Autodesk Inventor part; units mm, degrees
ref_plane "YZ Plane" through (0, 0, 0) normal (1, 0, 0) x (0, 1, 0)
ref_plane "XZ Plane" through (0, 0, 0) normal (0, 1, 0) x (-1, 0, 0)
ref_plane "XY Plane" through (0, 0, 0) normal (0, 0, 1) x (1, 0, 0)
sketch "Sketch1" plane through (0, 0, 0) normal (0, 1, 0) x (-1, 0, 0)
  line L0 (-15, -15) -> (15, -15)
  line L1 (15, -15) -> (15, 15)
  line L2 (15, 15) -> (-15, 15)
  line L3 (-15, 15) -> (-15, -15)
  line L4 (-15, -15) -> (15, 15) construction
  line L5 (15, -15) -> (-15, 15) construction
  point P0 (0, 0)
  dimension "d0" = 30
  dimension "d1" = 30
extrude "Extrusion1" add sketch "Sketch1" along normal blind 5
sketch "Sketch2" plane through (15, 0, 15) normal (1, 0, 0) x (0, 0, -1)
  line L0 (0, 5) -> (30, 5)
  line L1 (5, 4.05) -> (25, 4.05)
  line L2 (0, 0) -> (30, 0)
  line L3 (5, 4.6) -> (5, 4.05)
  line L4 (5, 4.6) -> (6, 4.6)
  line L5 (6, 4.6) -> (6, 5)
  line L6 (15, -1.7486) -> (15, 8.5822)
  line L7 (25, 4.05) -> (5, 4.05)
  line L8 (25, 4.6) -> (25, 4.05)
  line L9 (25, 4.6) -> (24, 4.6)
  line L10 (24, 4.6) -> (24, 5)
  point P0 (15, 0)
  point P1 (15, 0)
  point P2 (15, 0)
  dimension "d4" = 10
  dimension "d5" = 20
  dimension "d10" = 0.55
  dimension "d12" = 0.4
  dimension "d13" = 1
extrude "Extrusion2" cut sketch "Sketch2" against normal blind 25
sketch "Sketch3" plane through (0, 5, 0) normal (0, 1, 0) x (1, 0, 0)
  line L0 (-10, 9) -> (15, 9)
  line L1 (15, -9) -> (-10, -9)
  line L2 (-10, 9) -> (-7.5, 9)
  line L3 (-7.5, 9) -> (-7.5, -9)
  line L4 (-7.5, -9) -> (-10, -9)
  line L5 (-10, -9) -> (-10, 9)
  line L6 (-7.5, -1) -> (-10, -1)
  line L7 (-10, -1) -> (-10, 1)
  line L8 (-10, 1) -> (-7.5, 1)
  line L9 (-7.5, 1) -> (-7.5, -1)
  point P0 (0, 0)
  dimension "d16" = 2.5
  dimension "d17" = 2
  dimension "d18" = 1
extrude "Extrusion3" add sketch "Sketch3" against normal up to surface (0.4 mm away) contours L0 L3 L8 L5 | L6 L3 L1 L5
fillet "Fillet1" radius 1 6 edges at (15, 4.8, 9) (15, 4.8, -9) (-7.5, 4.8, -1) (-7.5, 4.8, 1) (-7.5, 4.8, 9) (-7.5, 4.8, -9)
sketch "Sketch4" plane through (0, 5, 0) normal (0, 1, 0) x (1, 0, 0)
  point P0 (0, 0)
  point P1 (12.5, -12.5)
  point P2 (-12.5, -12.5)
  point P3 (-12.5, 12.5)
  point P4 (12.5, 12.5)
  dimension "d22" = 25
  dimension "d23" = 12.5
  dimension "d24" = 25
  dimension "d25" = 12.5
hole "Hole1" at (12.5, 5, 12.5) at (-12.5, 5, 12.5) at (-12.5, 5, -12.5) at (12.5, 5, -12.5) direction (0, -1, 0) diameter 2 end through all
properties part number "Flex Circuit Slot"
For this review, take the finished solid that the model builds, in its own axes (mm). A direction names the side the tool comes from. Round coordinates to 2 decimals unless told otherwise and drop trailing zeros. Write each loop counter-clockwise with the first axis right and the second up, starting at its lowest first coordinate (ties: lowest second). Pieces come first, ordered by that corner, then holes. Notation, with made-up numbers: (6.25, 6.5) - (37.25, 6.5) arc R13 ccw to (37.25, 22.5) - close; hole circle Ø7 at (87, -14). An arc over 180 degrees is marked (long way). Use a Markdown table: item, result.
Q1. We need section A-A (x = -12.5). Give the boundary of the cut face in (y, z).
Derived:
| item | result |
|---|---|
| outline | (0, -15) - (5, -15) - (5, -13.5) - (0, -13.5) - close; (0, -11.5) - (5, -11.5) - (5, 11.5) - (0, 11.5) - close; (0, 13.5) - (5, 13.5) - (5, 15) - (0, 15) - close |
Q2. Wall thickness on line 1 along X through (y, z) = (3.3, 12.5); line 2 along Z through (x, y) = (-4.75, 4.25): over which ranges is each line inside the solid? List them lowest first.
Derived:
| item | result |
|---|---|
| line 1 | x = -15 to -13.5, -11.5 to 11.5, 13.5 to 15 |
| line 2 | z = -15 to -10, 10 to 15 |
Q3. We need section B-B (z = 3.25). Give the boundary of the cut face in (x, y), plus the area to 3 significant figures.
Derived:
| item | result |
|---|---|
| outline | (-15, 0) - (15, 0) - (15, 4.05) - (-10, 4.05) - (-10, 4.6) - (-7.5, 4.6) - (-7.5, 5) - (-15, 5) - close |
| area | 127 mm2 |
Q4. The part is to be moulded in two halves that separate along Z. For faces 1 (the flat face through (-10, 5, 4)), 2 (the flat face through (0, 2, 15)), 3 (the cylindrical face through (-7.199, 4.797, 8.715)), say which applies: pulls with the +Z half, pulls with the -Z half, needs draft (parallel to the pull), parting line crosses it, or undercut.
Derived:
| item | result |
|---|---|
| face 1 | needs draft |
| face 2 | pulls with the +Z half |
| face 3 | undercut |
Q5. Clearance check with a flat-ended pin moving along its axis: pin 1 (1 mm diameter, centred on x = 3.5, z = -2.5, fed in from +Y). State where the tip first meets the part, or that it passes through.
Derived:
| item | result |
|---|---|
| pin 1 | stops at y = 4.05 |
Q6. Machinability: for faces 4 (the flat face through (3, 4.05, 0)), 5 (the cylindrical face through (-7.215, 4.797, -8.699)), 6 (the flat face through (0, 0, 0)), which of the approach directions +Z, -Z, +X, -X, +Y, -Y give a long, thin tool a straight path to every point of the face, cutting with its end or side? Answer none if there is none.
Derived:
| item | result |
|---|---|
| face 4 | +X |
| face 5 | +X, +Y |
| face 6 | +Z, -Z, +X, -X, -Y |
Q7. We need section D-D (x = 1). Give the boundary of the cut face in (y, z).
Derived:
| item | result |
|---|---|
| outline | (0, -15) - (5, -15) - (5, -9) - (4.6, -9) - (4.6, -10) - (4.05, -10) - (4.05, 10) - (4.6, 10) - (4.6, 9) - (5, 9) - (5, 15) - (0, 15) - close |
Q8. We need section C-C (z = 12.5). Give the boundary of the cut face in (x, y), plus the area to 3 significant figures.
Derived:
| item | result |
|---|---|
| outline | (-15, 0) - (-13.5, 0) - (-13.5, 5) - (-15, 5) - close; (-11.5, 0) - (11.5, 0) - (11.5, 5) - (-11.5, 5) - close; (13.5, 0) - (15, 0) - (15, 5) - (13.5, 5) - close |
| area | 130 mm2 |
